Part model, mm, in its own coordinate system. Give positions to 0.01 mm unless a question says otherwise; leave off trailing zeros. Write each loop counter-clockwise with the first axis right and the second up, starting at its lowest first coordinate (ties: lowest second). Pieces come first, ordered by that corner, then holes.
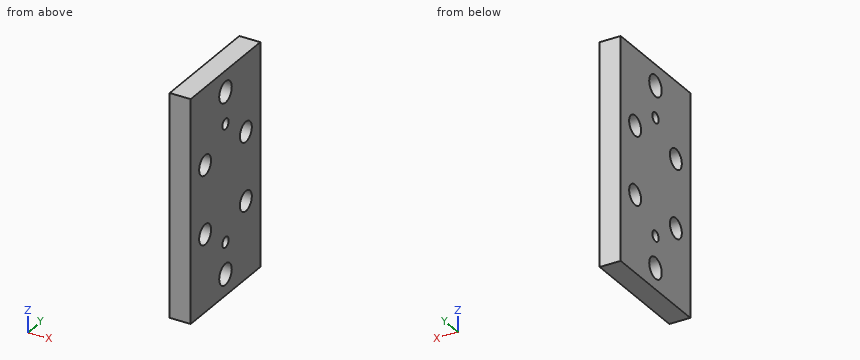
Autodesk Inventor part; units mm, degrees
ref_plane "YZ Plane" through (0, 0, 0) normal (1, 0, 0) x (0, 1, 0)
ref_plane "XZ Plane" through (0, 0, 0) normal (0, 1, 0) x (-1, 0, 0)
ref_plane "XY Plane" through (0, 0, 0) normal (0, 0, 1) x (1, 0, 0)
sketch "Sketch1" plane through (0, 0, 0) normal (1, 0, 0) x (0, 1, 0)
  line L0 (-6, -12.5) -> (-6, -12.9)
  arc A0 (-6, -12.9) -> (-5.6, -13.3) centre (-5.6, -12.9) ccw
  line L1 (-5.6, -13.3) -> (-4.9, -13.3)
  arc A1 (-4.9, -13.3) -> (-4.7, -13.1) centre (-4.9, -13.1) ccw
  line L2 (-4.7, -13.1) -> (-4.7, -12.85)
  arc A2 (-4.5, -12.65) -> (-4.7, -12.85) centre (-4.5, -12.85) ccw
  line L3 (-4.5, -12.65) -> (-1.8, -12.65)
  arc A3 (-1.4, -13.05) -> (-1.8, -12.65) centre (-1.8, -13.05) ccw
  line L4 (-1.4, -13.05) -> (-1.4, -18.75)
  line L5 (-1.8, -19.15) -> (-4.5, -19.15)
  arc A4 (-1.8, -19.15) -> (-1.4, -18.75) centre (-1.8, -18.75) ccw
  arc A5 (-4.7, -18.95) -> (-4.5, -19.15) centre (-4.5, -18.95) ccw
  line L6 (-4.7, -18.95) -> (-4.7, -18.7)
  arc A6 (-4.7, -18.7) -> (-4.9, -18.5) centre (-4.9, -18.7) ccw
  line L7 (-4.9, -18.5) -> (-5.6, -18.5)
  arc A7 (-5.6, -18.5) -> (-6, -18.9) centre (-5.6, -18.9) ccw
  line L8 (-6, -18.9) -> (-6, -19.5)
  line L9 (-6.5, -6.5) -> (-6.5, -12.5)
  line L10 (-6.5, -12.5) -> (-2.5, -12.5)
  line L11 (-1.05, -19.5) -> (-6.5, -19.5)
  line L12 (-6.5, -19.5) -> (-6.5, -26)
  line L13 (-6.5, -26) -> (-1.05, -26)
  line L14 (-6, -26) -> (-6, -26.6)
  arc A8 (-6, -26.6) -> (-5.6, -27) centre (-5.6, -26.6) ccw
  line L15 (-5.6, -27) -> (-4.9, -27)
  arc A9 (-4.9, -27) -> (-4.7, -26.8) centre (-4.9, -26.8) ccw
  arc A10 (-4.5, -26.35) -> (-4.7, -26.55) centre (-4.5, -26.55) ccw
  line L16 (-4.7, -26.8) -> (-4.7, -26.55)
  line L17 (-4.5, -26.35) -> (-1.8, -26.35)
  arc A11 (-1.4, -26.75) -> (-1.8, -26.35) centre (-1.8, -26.75) ccw
  line L18 (-1.4, -26.75) -> (-1.4, -32.45)
  arc A12 (-1.8, -32.85) -> (-1.4, -32.45) centre (-1.8, -32.45) ccw
  line L19 (-1.8, -32.85) -> (-4.5, -32.85)
  arc A13 (-4.7, -32.65) -> (-4.5, -32.85) centre (-4.5, -32.65) ccw
  line L20 (-4.7, -32.65) -> (-4.7, -32.4)
  arc A14 (-4.7, -32.4) -> (-4.9, -32.2) centre (-4.9, -32.4) ccw
  line L21 (-4.9, -32.2) -> (-5.6, -32.2)
  arc A15 (-5.6, -32.2) -> (-6, -32.6) centre (-5.6, -32.6) ccw
  line L22 (-6, -32.6) -> (-6, -33)
  line L23 (-2.5, -33) -> (-6.5, -33)
  line L24 (-6.5, -33) -> (-6.5, -39)
  line L25 (32.5, 0) -> (0, 0)
  circle A16 centre (0, -6.5) radius 4.75
  circle A17 centre (32.5, -6.5) radius 4.75
  circle A18 centre (0, -39) radius 4.75
  circle A19 centre (32.5, -39) radius 4.75
  line L26 (39, -26) -> (39, -19.5)
  line L27 (39, -12.5) -> (39, -6.5)
  line L28 (39, -39) -> (39, -33)
  line L29 (26.5, -45.5) -> (32.5, -45.5)
  line L30 (0, -45.5) -> (6, -45.5)
  line L31 (13, -45.5) -> (19.5, -45.5)
  circle A20 centre (16.2588, 5.0016) radius 2.5
  circle A21 centre (16.25, -50.5) radius 2.5
  line L32 (44, 10) -> (-11.5, 10)
  line L33 (-11.5, 10) -> (-11.5, -55.5)
  line L34 (-11.5, -55.5) -> (44, -55.5)
  line L35 (44, -55.5) -> (44, 10)
  line L36 (44, 10) -> (-11.5, 10)
  line L37 (-11.5, 10) -> (-11.5, 30)
  line L38 (-11.5, 30) -> (44, 30)
  line L39 (44, 30) -> (44, 10)
  line L40 (44, -55.5) -> (-11.5, -55.5)
  line L41 (-11.5, -55.5) -> (-11.5, -75.5)
  line L42 (-11.5, -75.5) -> (44, -75.5)
  line L43 (44, -75.5) -> (44, -55.5)
  circle A22 centre (16.25, 20) radius 5
  circle A23 centre (16.25, -65.5) radius 5
  point P0 (24.75, -17.8425)
  point P1 (-11.5, 10)
  dimension "d0" = 20
  dimension "d1" = 20
  dimension "d2" = 10
  dimension "d3" = 10
extrude "Extrusion1" add sketch "Sketch1" along normal blind 10
properties part number "PlacaMediaHidráulicos_CPY"
1) Saw through at C-C, the plane z = -50.5. Write the cut outline in (x, y).
Answers follow:
outline: (0, -11.5) - (10, -11.5) - (10, 13.75) - (0, 13.75) - close; (0, 18.75) - (10, 18.75) - (10, 44) - (0, 44) - close
2) Pin check, flat tip, straight feed: pin 1 Ø5.5 at (y, z) = (0, -6.5) entering from +X. Stop position of the tip, or through.
Answers follow:
pin 1: passes through
3) Saw through at A-A, the plane z = -6.5. Write the cut outline in (x, y), then the cut area to 3 significant figures.
Answers follow:
outline: (0, -11.5) - (10, -11.5) - (10, -4.75) - (0, -4.75) - close; (0, 4.75) - (10, 4.75) - (10, 27.75) - (0, 27.75) - close; (0, 37.25) - (10, 37.25) - (10, 44) - (0, 44) - close
area: 365 mm2
4) Wall check: L1, parallel to Z at x = 7.75, y = 32.5; L2, parallel to Z at x = 1, y = 36.5; L3, parallel to Y at x = 1.75, z = -4. Give the ranges that are in metal, low to high.
Answers follow:
L1: z = -75.5 to -43.75, -34.25 to -11.25, -1.75 to 30
L2: z = -75.5 to -41.56, -36.44 to -9.06, -3.94 to 30
L3: y = -11.5 to -4.04, 4.04 to 28.46, 36.54 to 44
5) Saw through at D-D, the plane y = 16.25. Write the cut outline in (x, z), then the cut area to 3 significant figures.
Answers follow:
outline: (0, -75.5) - (10, -75.5) - (10, -70.5) - (0, -70.5) - close; (0, -60.5) - (10, -60.5) - (10, -53) - (0, -53) - close; (0, -48) - (10, -48) - (10, 2.5) - (0, 2.5) - close; (0, 7.5) - (10, 7.5) - (10, 15) - (0, 15) - close; (0, 25) - (10, 25) - (10, 30) - (0, 30) - close
area: 755 mm2
6) Saw through at B-B, the plane y = 32.5. Write the cut outline in (x, z).
Answers follow:
outline: (0, -75.5) - (10, -75.5) - (10, -43.75) - (0, -43.75) - close; (0, -34.25) - (10, -34.25) - (10, -11.25) - (0, -11.25) - close; (0, -1.75) - (10, -1.75) - (10, 30) - (0, 30) - close
